For this review, take the finished solid that the model builds, in its own axes (mm). Face numbers are marked on the shaded views. A direction names the side the tool comes from. Give positions to 0.01 mm unless a question says otherwise; leave off trailing zeros. Order: outer loops, then holes, each group sorted by start corner. A loop starts at its lowest first (then second) coordinate and runs counter-clockwise, first axis right, second up. Notation, with made-up numbers: M -38,-27.75 L -6,-27.75 A16 cw -6,-6.75 Z; hole C -15,41 d7. An arc over 180 degrees is marked long. Answer as CSV lines item,"result". Start each with the question number.
1. We need section C-C, the plane x = 22. Give the boundary of the cut face in (y, z), and give its area (3 significant figures).
2. We need section D-D, the plane x = 11.75. Give the boundary of the cut face in (y, z).
3. Machinability: for the marked faces 1, 2 and 3, which of the approach directions +Z, -Z, +X, -X, +Y, -Y give a long, thin tool a straight path to every point of the face, cutting with its end or side? Answer none if there is none.
4. We need section A-A, the plane y = 24. Give the boundary of the cut face in (x, z) (3 decimals).
5. We need section B-B, the plane y = 6.5. Give the boundary of the cut face in (x, z) (3 decimals), and give its area (3 significant figures).
6. Mouldability with a two-part tool opening along Y and no side actions: class the marked faces 4, 5 and 6 as pulls with the +Y half, pulls with the -Y half, needs draft (parallel to the pull), parting line crosses it, or undercut.
7. Clearance check with flat-ended pins moving along their axes: P1, Ø1.5, axis at x = 14.5, z = 12, coming from the -Y side; P2, Ø1, axis at x = 1.5, z = 10, coming from the +Y side; P3, Ø1, axis at y = 23, z = 6, coming from the +X side (3 decimals). State where each tip first meets the part, or that it passes through.
8. For line 1 along X through (y, z) = (1.75, 10); line 2 along X through (y, z) = (7, 1.5) (3 decimals); line 3 along Y through (x, z) = (10.5, 5), list the stretches that pass through material, from the lowest coordinate up.
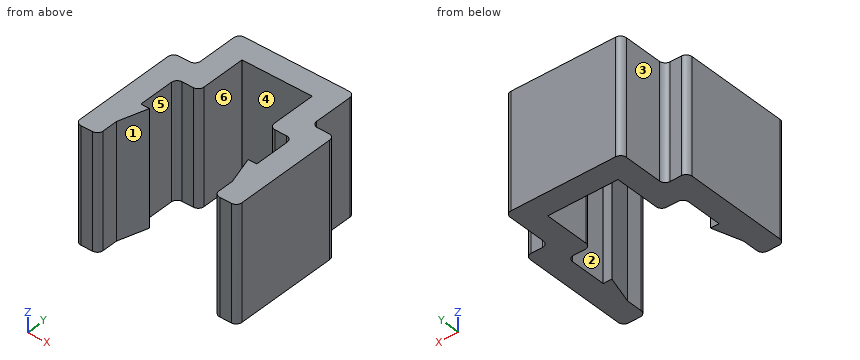
from build123d import *

# Parameters (mm, degrees)
F0_DEPTH = 20
F4_R     = 1
F2_DEPTH = 20


with BuildPart() as f0:
    # F3 (on Top) → F0 (new body)
    with BuildSketch(Plane.XY):
        Polygon((0, 20), (0, 0), (4, 0), (4, 16), (7.975, 16), (7.975, 24.8), (20.225, 24.8), (20.225, 16), (24.2, 16), (24.2, 0), (28.2, 0), (28.2, 20), (24.225, 20), (24.225, 28.8), (3.975, 28.8), (3.975, 20), align=None)
    extrude(amount=F0_DEPTH)

    # F4
    f4_edges = [f0.edges().sort_by_distance(p)[0] for p in [
        (4, 16, 10),
        (24.2, 16, 10),
        (7.975, 16, 10),
        (20.225, 16, 10),
        (0, 0, 10),
        (4, 0, 10),
        (24.2, 0, 10),
        (28.2, 0, 10),
        (0, 20, 10),
        (3.975, 28.8, 10),
        (3.975, 20, 10),
        (24.225, 28.8, 10),
        (24.225, 20, 10),
        (28.2, 20, 10),
    ]]
    fillet(f4_edges, radius=F4_R)

    # F1 (on face) → F2 (join)
    with BuildSketch(Plane.XY.offset(20)):
        Polygon((5.5, 8.75), (4, 8.75), (4, 3.75), align=None)
        Polygon((24.2, 3.75), (24.2, 8.75), (22.7, 8.75), align=None)
    extrude(amount=-F2_DEPTH)


solid = f0.part
Result set:
1,outline,"M 16,0 L 28.8,0 L 28.8,20 L 16,20 Z"
1,area,"256 mm2"
2,outline,"M 24.8,0 L 28.8,0 L 28.8,20 L 24.8,20 Z"
3,face 1,"+Z, -Z, -Y"
3,face 2,"+Z, -Z"
3,face 3,"+Z, -Z, -X, +Y"
4,outline,"M 3.975,0 L 7.975,0 L 7.975,20 L 3.975,20 Z; M 20.225,0 L 24.225,0 L 24.225,20 L 20.225,20 Z"
5,outline,"M 0,0 L 4.825,0 L 4.825,20 L 0,20 Z; M 23.375,0 L 28.2,0 L 28.2,20 L 23.375,20 Z"
5,area,"193 mm2"
6,face 4,"pulls with the -Y half"
6,face 5,"undercut"
6,face 6,"needs draft"
7,P1,"y = 24.8"
7,P2,"y = 20"
7,P3,"x = 24.225"
8,line 1,"0 to 4, 24.2 to 28.2"
8,line 2,"0 to 4.975, 23.225 to 28.2"
8,line 3,"24.8 to 28.8"
